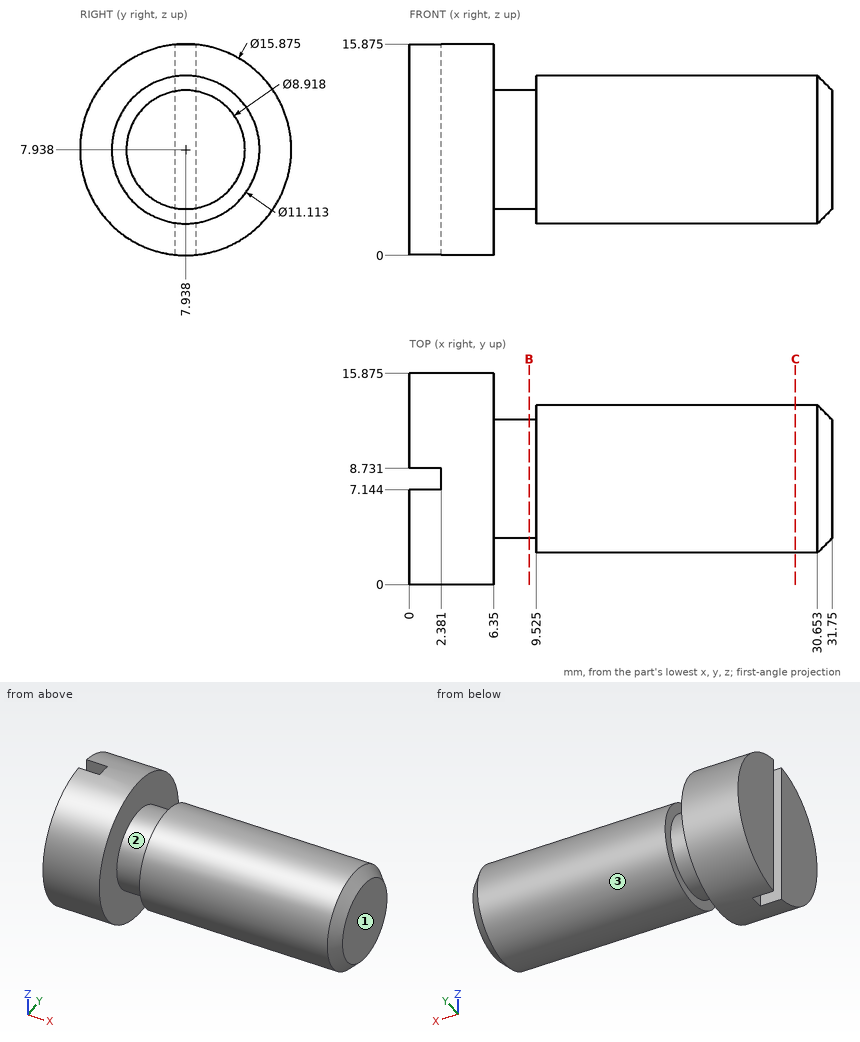
Study the drawing (mm; zero at the part's minimum x, y, z) and answer. A direction names the side the tool comes from. Give positions to 0.01 mm unless a question says otherwise; leave off trailing zeros. Loops run counter-clockwise (first coordinate to the right, second up) from the corner with the lowest first, then second, coordinate; pieces in that order, holes last. Notation, with made-up numbers: (-0.75, -23.5) -> (37.25, -23.5) arc R23 cw to (37.25, -11.5) -> close; hole circle Ø5 at (-21.5, -22). An arc over 180 degrees is marked (long way). Use a Markdown table: item, result. Add a question column.
1) Which of the six approach directions +Z, -Z, +X, -X, +Y, -Y give full straight-line access (tool end or side, diameter ignored) to the marked faces 1, 2 and 3?
2) Each of these flat-tipped pins is pushed along its axis until it touches: P1, Ø6, axis at x = 19.5, y = 5, coming from the +Z side; P2, Ø1.3, axis at y = 8, z = 11.5, coming from the -X side; P3, Ø3, axis at x = 27, z = 7, coming from the -Y side; P4, Ø1, axis at x = 7, y = 2.5, coming from the -Z side. Where does it stop, or does it pass through?
3) The part is cut by section C-C, the plane x = 29. Determine the outline of the cut face in (y, z), plus the area to 3 significant figures.
4) The part is cut by section B-B, the plane x = 9. Determine the outline of the cut face in (y, z).
5) Consider line 1 along Z through (x, y) = (12.5, 11.25) (1 decimal); line 2 along Z through (x, y) = (5, 2) (1 decimal); line 3 along Y through (x, z) = (20, 7.5). Determine where each line is inside the solid, lowest interval first.
Reported:
| question | item | result |
|---|---|---|
| 1 | face 1 | +Z, -Z, +X, +Y, -Y |
| 1 | face 2 | none |
| 1 | face 3 | +X |
| 2 | P1 | stops at z = 13.49 |
| 2 | P2 | stops at x = 2.38 |
| 2 | P3 | stops at y = 2.38 |
| 2 | P4 | passes through |
| 3 | outline | circle Ø11.11 at (7.94, 7.94) |
| 3 | area | 97.0 mm^2 |
| 4 | outline | circle Ø8.92 at (7.94, 7.94) |
| 5 | line 1 | z = 3.5 to 12.4 |
| 5 | line 2 | z = 2.7 to 13.2 |
| 5 | line 3 | y = 2.4 to 13.48 |
